```python
from build123d import *

# Parameters (mm, degrees)
BOSS_EXTRUDE1_DEPTH = 70
SKETCH2_R           = 25
CUT_EXTRUDE1_DEPTH  = 10
SKETCH5_R           = 25
CUT_EXTRUDE3_DEPTH  = 300
SKETCH6_R           = 5
CUT_EXTRUDE5_DEPTH  = 10


with BuildPart() as part:
    # Sketch1 → Boss-Extrude1 (new body)
    with BuildSketch(Plane(origin=(0, 0, 0), x_dir=(0, 0, -1), z_dir=(1, 0, 0))):
        Polygon((-93.245185093, 270.343761851), (0, 0), (-285.972750651, 0), (-285.972750651, -10), (14.027249349, -10), (-83.791705303, 273.604393673), align=None)
    extrude(amount=BOSS_EXTRUDE1_DEPTH)

    # Sketch2 → Cut-Extrude1 (cut)
    with BuildSketch(Plane(origin=(0, 3.260631822, -9.453479789), x_dir=(1, 0, 0), z_dir=(0, 0.3260631821748509, -0.945347978910417))):
        with Locations(Location((35, -185.972750651, 0), (0, 0, 270))):
            Circle(SKETCH2_R)
    extrude(amount=-CUT_EXTRUDE1_DEPTH, mode=Mode.SUBTRACT)

    # Sketch5 → Cut-Extrude3 (cut)
    with BuildSketch(Plane(origin=(0, 0, 0), x_dir=(1, 0, 0), z_dir=(0, 1, 0))):
        with Locations(Location((35, -225.972750651, 0), (0, 0, 270))):
            Circle(SKETCH5_R)
    extrude(amount=-CUT_EXTRUDE3_DEPTH, mode=Mode.SUBTRACT)

    # Sketch6 → Cut-Extrude5 (cut)
    with BuildSketch(Plane(origin=(0, 3.260631822, -9.453479789), x_dir=(1, 0, 0), z_dir=(0, 0.326063182174851, -0.945347978910417))):
        with Locations((50, -197.679491924)):
            Circle(SKETCH6_R)
        with Locations((20, -197.679491924)):
            Circle(SKETCH6_R)
        with Locations(Location((20, -127.679491924, 0), (0, 0, 270))):
            Circle(SKETCH6_R)
        with Locations(Location((50, -127.679491924, 0), (0, 0, 270))):
            Circle(SKETCH6_R)
    extrude(amount=-CUT_EXTRUDE5_DEPTH, mode=Mode.SUBTRACT)


solid = part.part
```
Build history of the part. All positions in model axes, mm. A direction names the side the tool comes from. Round coordinates to 2 decimals unless told otherwise and drop trailing zeros. Write each loop counter-clockwise with the first axis right and the second up, starting at its lowest first coordinate (ties: lowest second). Pieces come first, ordered by that corner, then holes. Notation, with made-up numbers: (39.5, -30) -> (69.5, -30) arc R7 ccw to (69.5, -22) -> close; hole circle Ø11 at (40, -20). An arc over 180 degrees is marked (long way). Put each result on its own line as item: value.
Item 1: Two-plate mould, pull along X, no slides. Class faces 1 (the face through (0, 80, 26)), 2 (the face through (35, -10, 138)), 3 (the face through (19.788, 158.707, 49.377)): pulls with the +X half, pulls with the -X half, needs draft (parallel to the pull), parting line crosses it, or undercut.
Here are the results:
face 1: pulls with the -X half
face 2: needs draft
face 3: undercut
Item 2: Flat gauge pins, fed straight in: P1, Ø8, axis at x = 18, y = 214.5, coming from the -Z side; P2, Ø12, axis at x = 40, y = 75, coming from the +Z side; P3, Ø5, axis at x = 15.5, z = 101.5, coming from the +Y side; P4, Ø2, axis at x = 52.5, z = 211.5, coming from the -Y side (3 decimals). Where does each tip first touch, or does it go through?
Here are the results:
P1: stops at z = 62.03
P2: stops at z = 27.94
P3: stops at y = 0
P4: passes through
Item 3: Slice it at A-A, the plane z = 207. Give the cut face in (x, y).
Here are the results:
outline: (0, -10) -> (18.72, -10) -> (18.72, 0) -> (0, 0) -> close; (51.28, -10) -> (70, -10) -> (70, 0) -> (51.28, 0) -> close
Item 4: Slice it at B-B, the plane x = 29. Give the cut face in (y, z), plus the area to 3 significant figures.
Here are the results:
outline: (-10, -14.03) -> (156.13, 43.27) -> (152.87, 52.73) -> (0, 0) -> (0, 201.7) -> (-10, 201.7) -> close; (-10, 250.24) -> (0, 250.24) -> (0, 285.97) -> (-10, 285.97) -> close; (198.75, 68.55) -> (202.01, 59.1) -> (273.6, 83.79) -> (270.34, 93.25) -> close
area: 4,890 mm^2
Item 5: Wall check: probe 1 along Y at (x, z) = (63, 223); probe 2 along Z at (x, y) = (64.5, 65.5); probe 3 along Z at (x, y) = (16, 226.5). Give the ranges that are in metal, low to high. Write a range as from..to.
Here are the results:
probe 1: y = -10..0
probe 2: z = 12.01..22.59
probe 3: z = 67.54..78.12
Item 6: Slice it at D-D, the plane y = 86.5. Give the cut face in (x, z) (3 decimals).
Here are the results:
outline: (0, 19.257) -> (70, 19.257) -> (70, 29.835) -> (0, 29.835) -> close
Item 7: Slice it at C-C, the plane z = 142. Give the cut face in (x, y), plus the area to 3 significant figures.
Here are the results:
outline: (0, -10) -> (70, -10) -> (70, 0) -> (0, 0) -> close
area: 700 mm^2
Item 8: Tool access for faces 4 (the face through (34.51, 137.064, 47.275)), 5 (the face through (54.216, 124.896, 37.715)): list every direction of +Z, -Z, +X, -X, +Y, -Y with a clear straight run to the whole face (end or side of a thin tool).
Here are the results:
face 4: +Z, +X, -X
face 5: none
